from build123d import *

# Parameters (mm, degrees)
SKETCH1_R                = 20
BOSS_EXTRUDE1_DEPTH      = 5
SKETCH3_R                = 1
CUT_EXTRUDE2_DEPTH       = 10
CIRPATTERN1_COUNT        = 8
SKETCH5_R                = 6
BOSS_EXTRUDE3_DEPTH      = 3
CUT_EXTRUDE5_DEPTH       = 30.393876913
BOSS_EXTRUDE4_DEPTH      = 0.5
BOSS_EXTRUDE4_DEPTH_BACK = 4.96
SKETCH4_R                = 4.5
SKETCH10_R               = 3
CUT_EXTRUDE6_DEPTH       = 2
SKETCH11_R               = 1.5
CUT_EXTRUDE7_DEPTH       = 30.021543722


with BuildPart() as part:
    # Sketch1 → Boss-Extrude1 (new body)
    with BuildSketch(Plane(origin=(0, 0, 0), x_dir=(1, 0, 0), z_dir=(0, 1, 0))):
        with Locations(Location((0, 0, 0), (0, 0, 270))):
            Circle(SKETCH1_R)
    extrude(amount=BOSS_EXTRUDE1_DEPTH)

    # Sketch3 → Cut-Extrude2 (cut)
    with BuildSketch(Plane(origin=(0, 5, 0), x_dir=(1, 0, 0), z_dir=(0, 1, 0))):
        with Locations(Location((0, 15, 0), (0, 0, 270))):
            Circle(SKETCH3_R)
        with Locations(Location((0, 10, 0), (0, 0, 270))):
            Circle(SKETCH3_R)
    cut_extrude2 = extrude(amount=-CUT_EXTRUDE2_DEPTH, mode=Mode.SUBTRACT)

    # CirPattern1: Cut-Extrude2 ×8 about axis
    cirpattern1_axis = Axis((0, 0, 0), (0, 1, 0))
    for i in range(1, CIRPATTERN1_COUNT):
        add(cut_extrude2.rotate(cirpattern1_axis, i * 360 / CIRPATTERN1_COUNT), mode=Mode.SUBTRACT)

    # Sketch5 → Boss-Extrude3 (add)
    with BuildSketch(Plane.XZ):
        with Locations(Location((0, 0, 0), (0, 0, 90))):
            Circle(SKETCH5_R)
    extrude(amount=BOSS_EXTRUDE3_DEPTH)

    # Sketch8 → Cut-Extrude5 (cut, through all)
    with BuildSketch(Plane.XZ.offset(3)):
        with BuildLine():
            Line((0.7, 3.684087404), (0, 3.05))
            Line((0, 3.05), (-0.7, 3.684087404))
            ThreePointArc((-0.7, 3.684087404), (-0.779668841, 3.668053503), (-0.858971523, 3.650296964))
            Line((-0.858971523, 3.650296964), (-1.240546761, 2.786313646))
            Line((-1.240546761, 2.786313646), (-2.137935164, 3.080865663))
            ThreePointArc((-2.137935164, 3.080865663), (-2.204194696, 3.033813729), (-2.269419066, 2.985337016))
            Line((-2.269419066, 2.985337016), (-2.266591718, 2.040848349))
            Line((-2.266591718, 2.040848349), (-3.206201915, 1.944934261))
            ThreePointArc((-3.206201915, 1.944934261), (-3.247595264, 1.875), (-3.287463436, 1.804185178))
            Line((-3.287463436, 1.804185178), (-2.900722375, 0.942501833))
            Line((-2.900722375, 0.942501833), (-3.720087228, 0.472706055))
            ThreePointArc((-3.720087228, 0.472706055), (-3.729457108, 0.391981737), (-3.737075512, 0.311073332))
            Line((-3.737075512, 0.311073332), (-3.033291781, -0.318811813))
            Line((-3.033291781, -0.318811813), (-3.590735663, -1.081257322))
            ThreePointArc((-3.590735663, -1.081257322), (-3.566461936, -1.158813729), (-3.540513282, -1.235825919))
            Line((-3.540513282, -1.235825919), (-2.641377482, -1.525))
            Line((-2.641377482, -1.525), (-2.840513282, -2.448261485))
            ThreePointArc((-2.840513282, -2.448261485), (-2.786793096, -2.509239774), (-2.73176414, -2.569039642))
            Line((-2.73176414, -2.569039642), (-1.792745019, -2.467501833))
            Line((-1.792745019, -2.467501833), (-1.599140348, -3.391938995))
            ThreePointArc((-1.599140348, -3.391938995), (-1.525262412, -3.425795466), (-1.450668162, -3.458043072))
            Line((-1.450668162, -3.458043072), (-0.634130657, -2.983350182))
            Line((-0.634130657, -2.983350182), (-0.081261521, -3.749119439))
            ThreePointArc((-0.081261521, -3.749119439), (0, -3.75), (0.081261521, -3.749119439))
            Line((0.081261521, -3.749119439), (0.634130657, -2.983350182))
            Line((0.634130657, -2.983350182), (1.450668162, -3.458043072))
            ThreePointArc((1.450668162, -3.458043072), (1.525262412, -3.425795466), (1.599140348, -3.391938995))
            Line((1.599140348, -3.391938995), (1.792745019, -2.467501833))
            Line((1.792745019, -2.467501833), (2.73176414, -2.569039642))
            ThreePointArc((2.73176414, -2.569039642), (2.786793096, -2.509239774), (2.840513282, -2.448261485))
            Line((2.840513282, -2.448261485), (2.641377482, -1.525))
            Line((2.641377482, -1.525), (3.540513282, -1.235825919))
            ThreePointArc((3.540513282, -1.235825919), (3.566461936, -1.158813729), (3.590735663, -1.081257322))
            Line((3.590735663, -1.081257322), (3.033291781, -0.318811813))
            Line((3.033291781, -0.318811813), (3.737075512, 0.311073332))
            ThreePointArc((3.737075512, 0.311073332), (3.729457108, 0.391981737), (3.720087228, 0.472706055))
            Line((3.720087228, 0.472706055), (2.900722375, 0.942501833))
            Line((2.900722375, 0.942501833), (3.287463436, 1.804185178))
            ThreePointArc((3.287463436, 1.804185178), (3.247595264, 1.875), (3.206201915, 1.944934261))
            Line((3.206201915, 1.944934261), (2.266591718, 2.040848349))
            Line((2.266591718, 2.040848349), (2.269419066, 2.985337016))
            ThreePointArc((2.269419066, 2.985337016), (2.204194696, 3.033813729), (2.137935164, 3.080865663))
            Line((2.137935164, 3.080865663), (1.240546761, 2.786313646))
            Line((1.240546761, 2.786313646), (0.858971523, 3.650296964))
            ThreePointArc((0.858971523, 3.650296964), (0.779668841, 3.668053503), (0.7, 3.684087404))
        make_face()
    extrude(amount=-CUT_EXTRUDE5_DEPTH, mode=Mode.SUBTRACT)

    # Sketch4 → Boss-Extrude4 (add, two sides: drawn at the far end of the back side and taken through both)
    with BuildSketch(Plane(origin=(0, 5, 0), x_dir=(1, 0, 0), z_dir=(0, 1, 0)).offset(-BOSS_EXTRUDE4_DEPTH_BACK)):
        with Locations(Location((0, 0, 0), (0, 0, 270))):
            Circle(SKETCH4_R)
    extrude(amount=BOSS_EXTRUDE4_DEPTH + BOSS_EXTRUDE4_DEPTH_BACK)

    # Sketch10 → Cut-Extrude6 (cut)
    with BuildSketch(Plane(origin=(0, 5.5, 0), x_dir=(1, 0, 0), z_dir=(0, 1, 0))):
        with Locations(Location((0, 0, 0), (0, 0, 270))):
            Circle(SKETCH10_R)
    extrude(amount=-CUT_EXTRUDE6_DEPTH, mode=Mode.SUBTRACT)

    # Sketch11 → Cut-Extrude7 (cut, through all)
    with BuildSketch(Plane(origin=(0, 3.5, 0), x_dir=(1, 0, 0), z_dir=(0, 1, 0))):
        with Locations(Location((0, 0, 0), (0, 0, 270))):
            Circle(SKETCH11_R)
    extrude(amount=-CUT_EXTRUDE7_DEPTH, mode=Mode.SUBTRACT)


solid = part.part
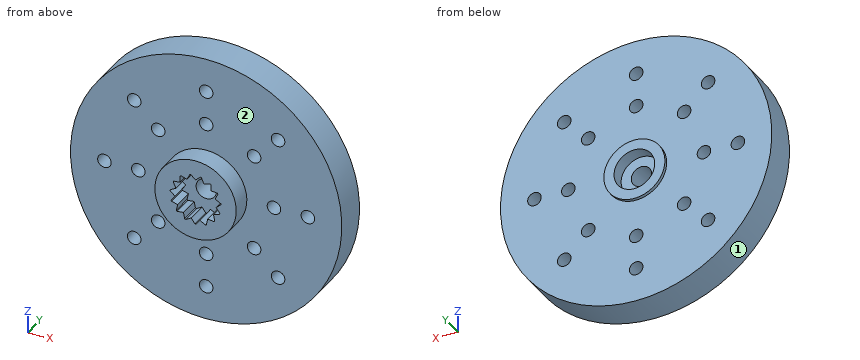
Design review of the part built by this model. Coordinates are the model's own, in mm. Face numbers are marked on the shaded views. A direction names the side the tool comes from. Give positions to 0.01 mm unless a question says otherwise; leave off trailing zeros. Write each loop counter-clockwise with the first axis right and the second up, starting at its lowest first coordinate (ties: lowest second). Pieces come first, ordered by that corner, then holes. Notation, with made-up numbers: M 67,-21 L 100,-21 A20 cw 100,-10 Z; hole C 58,16.5 d11. An arc over 180 degrees is marked long. Return JSON: item names as keys, results as strings. Group by question number.
Item 1: Take a section at C-C (z = -10.5). Give the boundary of the cut face in (x, y).
Item 2: Take a section at D-D (z = 13). Give the boundary of the cut face in (x, y), plus the area to 3 significant figures.
Item 3: Take a section at A-A (z = -15). Give the boundary of the cut face in (x, y), plus the area to 3 significant figures.
Item 4: Take a section at B-B (x = -15). Give the boundary of the cut face in (y, z), plus the area to 3 significant figures.
Item 5: Wall thickness on line 1 along Z through (x, y) = (-10.5, 4.5); line 2 along Y through (x, z) = (-11, -16); line 3 along Z through (x, y) = (1.5, -2): over which ranges is each line inside the solid? List them lowest first.
Item 6: Tool access review of the marked faces 1 and 2: name each direction out of +Z, -Z, +X, -X, +Y, -Y from which nothing blocks a thin tool from reaching the whole face with its end or side.
Item 7: Clearance check with flat-ended pins moving along their axes: pin 1 Ø2.5 at (x, z) = (7.07, -7.07) entering from +Y; pin 2 Ø3 at (y, z) = (-2, -8.5) entering from -X; pin 3 Ø1 at (x, y) = (-12.5, 3) entering from -Z; pin 4 Ø2.5 at (x, z) = (-7.07, -7.07) entering from -Y. State where each tip first meets the part, or that it passes through.
Return value:
{
 "1": {"outline": "M -17.02,0 L -11.6,0 L -11.6,5 L -17.02,5 Z; M -9.61,0 L -0.87,0 L -0.87,5 L -9.61,5 Z; M 0.87,0 L 9.61,0 L 9.61,5 L 0.87,5 Z; M 11.6,0 L 17.02,0 L 17.02,5 L 11.6,5 Z"},
 "2": {"outline": "M -15.2,0 L 15.2,0 L 15.2,5 L -15.2,5 Z", "area": "152 mm2"},
 "3": {"outline": "M -13.23,0 L -1,0 L -1,5 L -13.23,5 Z; M 1,0 L 13.23,0 L 13.23,5 L 1,5 Z", "area": "122 mm2"},
 "4": {"outline": "M 0,-13.23 L 5,-13.23 L 5,-1 L 0,-1 Z; M 0,1 L 5,1 L 5,13.23 L 0,13.23 Z", "area": "122 mm2"},
 "5": {"line 1": "z = -17.02 to -11.6, -9.61 to -0.87, 0.87 to 9.61, 11.6 to 17.02", "line 2": "y = 0 to 5", "line 3": "z = -5.81 to -3.44, 2.87 to 5.81"},
 "6": {"face 1": "+Y, -Y", "face 2": "-Y"},
 "7": {"pin 1": "stops at y = 5", "pin 2": "passes through", "pin 3": "stops at z = -16", "pin 4": "stops at y = 0"}
}
